Could you check a few things on this model? Use its own coordinates, in mm. Face numbers are marked on the shaded views. Give positions to 0.01 mm unless a question says otherwise; leave off trailing zeros. Loops run counter-clockwise (first coordinate to the right, second up) from the corner with the lowest first, then second, coordinate; pieces in that order, holes last. Notation, with made-up numbers: M 22,11.5 L 35,11.5 A15 cw 35,20.5 Z; hole C 4.5,86.25 d5. An arc over 180 degrees is marked long. Write each question's results on one line, items separated by ' | '. Start each with the question number.
from build123d import *

# Parameters (mm, degrees)
F0_R     = 48
F0_R_2   = 39.5
F0_R_3   = 5.3
F0_R_4   = 2.3
F1_DEPTH = 3
F2_DEPTH = 0.6


with BuildPart() as f1:
    # F0 (on Top) → F1 (new body)
    with BuildSketch(Plane.XY):
        Circle(F0_R)
        Circle(F0_R_2, mode=Mode.SUBTRACT)
        Circle(F0_R_3)
        Circle(F0_R_4, mode=Mode.SUBTRACT)
    extrude(amount=F1_DEPTH)

    # F0 (on Top) → F2 (join)
    with BuildSketch(Plane.XY):
        Circle(F0_R)
        Circle(F0_R_2, mode=Mode.SUBTRACT)
        Circle(F0_R_2)
        Circle(F0_R_3, mode=Mode.SUBTRACT)
        Circle(F0_R_3)
        Circle(F0_R_4, mode=Mode.SUBTRACT)
    extrude(amount=-F2_DEPTH)


solid = f1.part
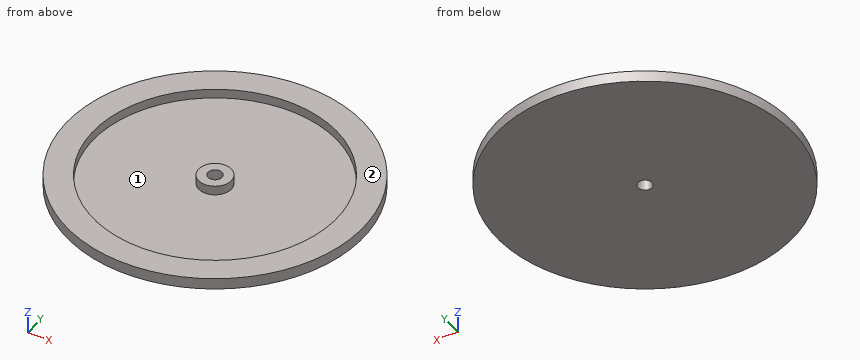
1) If we section it at A-A on y = 0: Write out the boundary of the cut face in (x, z), plus the area to 3 significant figures.
2) I'm going to push flat-ended pins straight in: P1, Ø1.5, axis at x = 14, z = 1.5, coming from the -Y side (3 decimals); P2, Ø1.5, axis at x = -29, z = 1, coming from the +Y side; P3, Ø2, axis at y = -12, z = 1, coming from the +X side. Where does each tip first touch, or does it pass through?
3) Please list where these lines run through material, in increasing order: line 1 (Y direction, x = 0, z = 1.8); line 2 (X direction, y = 1.5, z = 2.45); line 3 (Z direction, x = -20.5, y = 29). Write a range as from..to.
4) If we section it at D-D on y = 13: Write out the boundary of the cut face in (x, z).
5) If we section it at C-C on z = 0.8: Write out the boundary of the cut face in (x, y), plus the area to 3 significant figures.
6) Thinking about a two-plate mould opening in Y: for the marked faces 1 and 2, which applies, pulls with the +Y half, pulls with the -Y half, needs draft (parallel to the pull), parting line crosses it, or undercut?
Calculated:
1) outline: M -48,-0.6 L -2.3,-0.6 L -2.3,3 L -5.3,3 L -5.3,0 L -39.5,0 L -39.5,3 L -48,3 Z; M 2.3,-0.6 L 48,-0.6 L 48,3 L 39.5,3 L 39.5,0 L 5.3,0 L 5.3,3 L 2.3,3 Z | area: 124 mm2
2) P1: stops at y = -46.135 | P2: stops at y = 38.81 | P3: stops at x = 46.72
3) line 1: y = -48..-39.5, -5.3..-2.3, 2.3..5.3, 39.5..48 | line 2: x = -47.98..-39.47, -5.08..-1.74, 1.74..5.08, 39.47..47.98 | line 3: z = -0.6..0
4) outline: M -46.21,-0.6 L 46.21,-0.6 L 46.21,3 L 37.3,3 L 37.3,0 L -37.3,0 L -37.3,3 L -46.21,3 Z
5) outline: C 0,0 d96; C 0,0 d10.6; hole C 0,0 d79; hole C 0,0 d4.6 | area: 2,410 mm2
6) face 1: undercut | face 2: needs draft
